```python
from build123d import *

# Parameters (mm, degrees)
SKETCH1_W           = 190
SKETCH1_H           = 80
BOSS_EXTRUDE1_DEPTH = 10
CUT_EXTRUDE1_DEPTH  = 10
FILLET1_R           = 5


with BuildPart() as part:
    # Sketch1 → Boss-Extrude1 (new body)
    with BuildSketch(Plane.XY):
        Rectangle(SKETCH1_W, SKETCH1_H)
    extrude(amount=BOSS_EXTRUDE1_DEPTH)

    # Sketch2 → Cut-Extrude1 (cut)
    with BuildSketch(Plane.XY):
        Polygon((-75, -30), (-85, -30), (-85, 30), (-75, 30), (-75, 6), (-61, 6), (-61, 30), (-51, 30), (-51, -30), (-61, -30), (-61, -4), (-75, -4), align=None)
        Polygon((-31, 20), (-31, 6), (-7, 6), (-7, -6), (-31, -6), (-31, -20), (-7, -20), (-7, -30), (-41, -30), (-41, 30), (-7, 30), (-7, 20), align=None)
        Polygon((43, -30), (33, -30), (33, 20), (23, 6.666666667), (13, 20), (13, -30), (3, -30), (3, 30), (13, 30), (23, 16.666666667), (33, 30), (43, 30), align=None)
        with BuildLine():
            Line((53, -12), (53, 30))
            Line((53, 30), (63, 30))
            Line((63, 30), (63, -13))
            ThreePointArc((63, -13), (69, -19), (75, -13))
            Line((75, -13), (75, 30))
            Line((75, 30), (85, 30))
            Line((85, 30), (85, -12))
            ThreePointArc((85, -12), (69, -29.031219542), (53, -12))
        make_face()
    extrude(amount=CUT_EXTRUDE1_DEPTH, mode=Mode.SUBTRACT)

    # Fillet1
    fillet1_edges = [part.edges().sort_by_distance(p)[0] for p in [
        (63, 30, 5),
        (53, 30, 5),
        (85, 30, 5),
        (75, 30, 5),
        (-85, -30, 5),
        (-75, -30, 5),
        (-75, -4, 5),
        (-61, -4, 5),
        (-61, -30, 5),
        (-51, -30, 5),
        (-51, 30, 5),
        (-61, 30, 5),
        (-61, 6, 5),
        (-75, 6, 5),
        (-75, 30, 5),
        (-85, 30, 5),
        (-31, 20, 5),
        (-7, 20, 5),
        (-7, 30, 5),
        (-41, 30, 5),
        (-41, -30, 5),
        (-7, -30, 5),
        (-7, -20, 5),
        (-31, -20, 5),
        (-31, -6, 5),
        (-7, -6, 5),
        (-7, 6, 5),
        (-31, 6, 5),
        (13, 20, 5),
        (33, 20, 5),
        (33, -30, 5),
        (43, -30, 5),
        (43, 30, 5),
        (33, 30, 5),
        (23, 16.666666667, 5),
        (13, 30, 5),
        (3, 30, 5),
        (3, -30, 5),
        (13, -30, 5),
    ]]
    fillet(fillet1_edges, radius=FILLET1_R - 0.0001)  # a hair under: the kernel refuses the full size


solid = part.part
```
Input: part model. Units: mm. Frame: model coordinates. Give positions to 0.01 mm unless a question says otherwise; leave off trailing zeros. Order: outer loops, then holes, each group sorted by start corner. A loop starts at its lowest first (then second) coordinate and runs counter-clockwise, first axis right, second up. Notation, with made-up numbers: M -27.5,32.25 L 19.5,32.25 A28 cw 19.5,62.25 Z; hole C 69,5.25 d1. An arc over 180 degrees is marked long. Return JSON: item names as keys, results as strings.
Item 1: Cut plane B-B (z = 6.75). State how many separate pieces and enclosed holes the cut face has, then the cut area to 3 significant figures.
Solutions:
{"separate pieces": "1", "enclosed holes": "4", "area": "9,890 mm^2"}
Item 2: Ray query, probe 1 along Y at (x, z) = (-26, 5.5); probe 2 along Y at (x, z) = (8, 7); probe 3 along Y at (x, z) = (-10, 9.25). Return the intervals inside material, ascending.
Solutions:
{"probe 1": "-40 to -30, -20 to -6, 6 to 20, 30 to 40", "probe 2": "-40 to -30, 30 to 40", "probe 3": "-40 to -29.58, -20.42 to -5.58, 5.58 to 20.42, 29.58 to 40"}
Item 3: Pull-direction query (Y, two-part tool) for faces 1 (the flat face through (-1, -40, 5)), 2 (the cylindrical face through (-76, 28, 5)), 3 (the flat face through (3, 0, 5)), 4 (the flat face through (95, -1, 5)); classes: +Y half, -Y half, draft (parallel to the pull), parting line (faces both ways), or undercut.
Solutions:
{"face 1": "-Y half", "face 2": "undercut", "face 3": "undercut", "face 4": "draft"}
Item 4: Cut plane A-A (x = 69). Return loops of the section in (y, z).
Solutions:
{"outline": "M -40,0 L -29.03,0 L -29.03,10 L -40,10 Z; M -19,0 L 40,0 L 40,10 L -19,10 Z"}
Item 5: First-contact query: P1, Ø2, axis at x = 67.5, y = 31, coming from the -Z side. Flat tip, straight axial feed; report the tip coordinate or a pass-through.
Solutions:
{"P1": "z = 0"}
